from build123d import *

# Parameters (mm, degrees)
F1_DEPTH = 30
F2_R     = 12.5
F3_DEPTH = 15
F4_DEPTH = 30
F5_R     = 8.5
F6_DEPTH = 15


with BuildPart() as f1:
    # F0 (on Top) → F1 (new body)
    with BuildSketch(Plane.XY):
        Polygon((-5, 8.6602540378), (-10, 0), (-5, -8.6602540378), (5, -8.6602540378), (10, 0), (5, 8.6602540378), align=None)
    extrude(amount=F1_DEPTH)

    # F2 (on face) → F3 (join)
    with BuildSketch(Plane.XY.offset(30)):
        Circle(F2_R)
        Polygon((-10, 0), (-5, 8.6602540378), (5, 8.6602540378), (10, 0), (5, -8.6602540378), (-5, -8.6602540378), align=None, mode=Mode.SUBTRACT)
    extrude(amount=F3_DEPTH)

    # F4 (add): a face of the model
    f4_faces = [f1.faces().sort_by_distance(p)[0] for p in [
        (0, 0, 30),
    ]]
    extrude(f4_faces, amount=F4_DEPTH)

    # F5 (on face) → F6 (join)
    with BuildSketch(Plane(origin=(0, 0, 0), x_dir=(1, 0, 0), z_dir=(0, 0, -1))):
        Circle(F5_R)
    extrude(amount=F6_DEPTH)


solid = f1.part
For this review, take the finished solid that the model builds, in its own axes (mm). A direction names the side the tool comes from. Coordinates: 2 decimals unless noted, no trailing zeros. Order: outer loops, then holes, each group sorted by start corner. A loop starts at its lowest first (then second) coordinate and runs counter-clockwise, first axis right, second up. Notation, with made-up numbers: (-37.5, 50) - (-33.5, 50) arc R22 cw to (-33.5, 62) - close; hole circle Ø6 at (34, 72.25). An arc over 180 degrees is marked (long way). Use one line per item in the form item = value.
Q1. For probe 1 along Z at (x, y) = (7.5, 7.5); probe 2 along Y at (x, z) = (-2.75, 19); probe 3 along X at (y, z) = (-7.5, 44), list the stretches that pass through material, from the lowest coordinate up. Write a range as from..to.
Checked values:
probe_1 = 30..45
probe_2 = -8.66..8.66
probe_3 = -10..10
Q2. Consider section A-A (x = 0). Give the boundary of the cut face in (y, z), then the cut area to 3 significant figures.
Checked values:
outline = (-12.5, 30) - (-8.66, 30) - (-8.66, 0) - (-8.5, 0) - (-8.5, -15) - (8.5, -15) - (8.5, 0) - (8.66, 0) - (8.66, 30) - (12.5, 30) - (12.5, 45) - (8.66, 45) - (8.66, 60) - (-8.66, 60) - (-8.66, 45) - (-12.5, 45) - close
area = 1,410 mm2
Q3. Consider section C-C (z = 13.5). Give the boundary of the cut face in (x, y), then the cut area to 3 significant figures.
Checked values:
outline = (-10, 0) - (-5, -8.66) - (5, -8.66) - (10, 0) - (5, 8.66) - (-5, 8.66) - close
area = 260 mm2
Q4. Consider section D-D (y = -10.25). Give the boundary of the cut face in (x, z).
Checked values:
outline = (-7.15, 30) - (7.15, 30) - (7.15, 45) - (-7.15, 45) - close
Q5. Consider section B-B (y = -3). Give the boundary of the cut face in (x, z), then the cut area to 3 significant figures.
Checked values:
outline = (-12.13, 30) - (-8.27, 30) - (-8.27, 0) - (-7.95, 0) - (-7.95, -15) - (7.95, -15) - (7.95, 0) - (8.27, 0) - (8.27, 30) - (12.13, 30) - (12.13, 45) - (8.27, 45) - (8.27, 60) - (-8.27, 60) - (-8.27, 45) - (-12.13, 45) - close
area = 1,350 mm2
Q6. For P1, Ø1, axis at y = -8, z = 11.5, coming from the -X side; P2, Ø3, axis at x = -6, z = 5, coming from the +Y side; P3, Ø5, axis at x = -1.5, z = 20.5, coming from the -Y side; P4, Ø4, axis at x = 1.5, y = -9, coming from the -Z side, all flat-tipped, find the tip position at first contact; note any pin that passes through.
Checked values:
P1 = -5.67
P2 = 8.66
P3 = -8.66
P4 = -15
Q7. For faces 1 (the cylindrical face through (4.57, -7.167, -7.395)), 2 (the flat face through (-7.465, 4.391, 14.79)), 3 (the flat face through (0, -8.66, 15)), 4 (the flat face through (-9, -3, 45)), list the 3-axis set-ups (+Z, -Z, +X, -X, +Y, -Y) from which the entire face can be reached by the end or side of a thin tool; tool diameter is ignored.
Checked values:
face_1 = -Z
face_2 = -Z, -X, +Y
face_3 = -Z, +X, -X, -Y
face_4 = +Z
